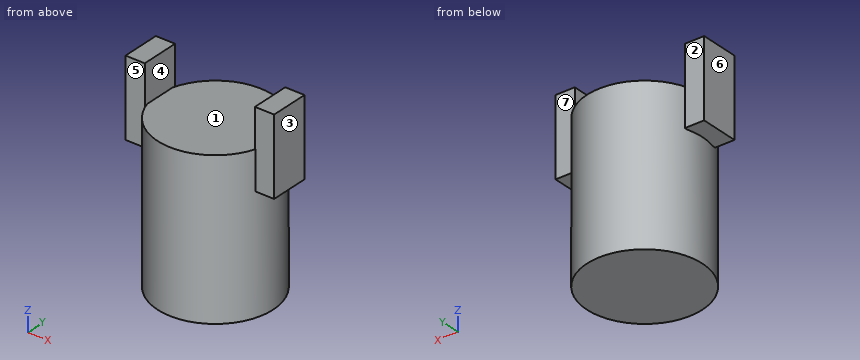
```python
from build123d import *

# Parameters (mm, degrees)
F0_R     = 38.1
F1_DEPTH = 101.6
F2_W     = 12.7
F2_H     = 25.4
F3_DEPTH = 25.4


# Not quite as in the source:
# - a feature of the source that left no trace in its solid (it failed there, or was rolled back) is left out


with BuildPart() as f1:
    # F0 (on Top) → F1 (new body)
    with BuildSketch(Plane.XY):
        Circle(F0_R)
    extrude(amount=F1_DEPTH)

    # F2 (on face) → F3 (join, symmetric)
    with BuildSketch(Plane.XY.offset(101.6)):
        with Locations((-42.9418016334, 0.0489659142)):
            Rectangle(F2_W, F2_H)
        with Locations((42.1098351814, 0.4470220127)):
            Rectangle(F2_W, F2_H)
    extrude(amount=F3_DEPTH, both=True)


solid = f1.part
```
Input: part model. Units: mm. Frame: model coordinates. Face numbers are marked on the shaded views. A direction names the side the tool comes from. Coordinates: 2 decimals unless noted, no trailing zeros. Write each loop counter-clockwise with the first axis right and the second up, starting at its lowest first coordinate (ties: lowest second). Pieces come first, ordered by that corner, then holes. Notation, with made-up numbers: (25, 3.25) - (69, 3.25) arc R11 ccw to (69, 20.25) - close; hole circle Ø8 at (4.5, 70.25). An arc over 180 degrees is marked (long way). Put each result on its own line as item: value. Start each with the question number.
1) Mould query, pull axis X, two halves, no side actions, for the marked faces 1, 2, 3 and 4. Classes: pulls with the +X half, pulls with the -X half, needs draft (parallel to the pull), parting line crosses it, or undercut.
2) Cut plane B-B (y = 0). Return the cut outline in (x, z).
3) Ray query, L1, parallel to Z at x = 30, y = -0.5; L2, parallel to X at y = -10.5, z = 111; L3, parallel to Y at x = -25, z = 97. Return the intervals inside material, ascending.
4) Cut plane D-D (z = 99). Return the cut outline in (x, y).
5) Reachability of the marked faces 5, 6 and 7 from +Z, -Z, +X, -X, +Y, -Y: full face, straight path, thin tool, end or side. Return the list, or none.
6) Cut plane C-C (x = 0). Return the cut outline in (y, z).
7) Contact query for flat-ended pins moving along their axis: pin 1 (8 mm diameter, centred on x = -22.5, z = 94.5, fed in from -Y); pin 2 (6.5 mm diameter, centred on x = -41.5, z = 111, fed in from +Y); pin 3 (14 mm diameter, centred on x = 43, y = -4, fed in from -Z); pin 4 (10 mm diameter, centred on y = -24.5, z = 59, fed in from +X). Output: stop coordinate, or through.
8) Cut plane A-A (z = 115.5). Return the cut outline in (x, y), plus the area to 3 significant figures.
Resolved:
1. face 1: undercut
1. face 2: needs draft
1. face 3: pulls with the +X half
1. face 4: undercut
2. outline: (-49.29, 76.2) - (-38.1, 76.2) - (-38.1, 0) - (38.1, 0) - (38.1, 76.2) - (48.46, 76.2) - (48.46, 127) - (35.76, 127) - (35.76, 101.6) - (-36.59, 101.6) - (-36.59, 127) - (-49.29, 127) - close
3. L1: z = 0 to 101.6
3. L2: x = -49.29 to -36.59, 35.76 to 48.46
3. L3: y = -28.75 to 28.75
4. outline: (-49.29, -12.65) - (-36.59, -12.65) - (-36.59, -10.61) arc R38.1 ccw to (36.08, -12.25) - (48.46, -12.25) - (48.46, 13.15) - (35.76, 13.15) arc R38.1 ccw to (-36.59, 10.61) - (-36.59, 12.75) - (-49.29, 12.75) - close
5. face 5: +Z, -Z, -X, -Y
5. face 6: +Z, -Z, -X, +Y, -Y
5. face 7: +Z, -Z, +X, +Y
6. outline: (-38.1, 0) - (38.1, 0) - (38.1, 101.6) - (-38.1, 101.6) - close
7. pin 1: stops at y = -33.31
7. pin 2: stops at y = 12.75
7. pin 3: stops at z = 0
7. pin 4: stops at x = 32.73
8. outline: (-49.29, -12.65) - (-36.59, -12.65) - (-36.59, 12.75) - (-49.29, 12.75) - close; (35.76, -12.25) - (48.46, -12.25) - (48.46, 13.15) - (35.76, 13.15) - close
8. area: 645 mm2
